Geometry: see drawing. Coordinates: mm, zero at the bounding-box minimum. A direction names the side the tool comes from. Round coordinates to 2 decimals unless told otherwise and drop trailing zeros. Write each loop counter-clockwise with the first axis right and the second up, starting at its lowest first coordinate (ties: lowest second). Pieces come first, ordered by that corner, then holes.
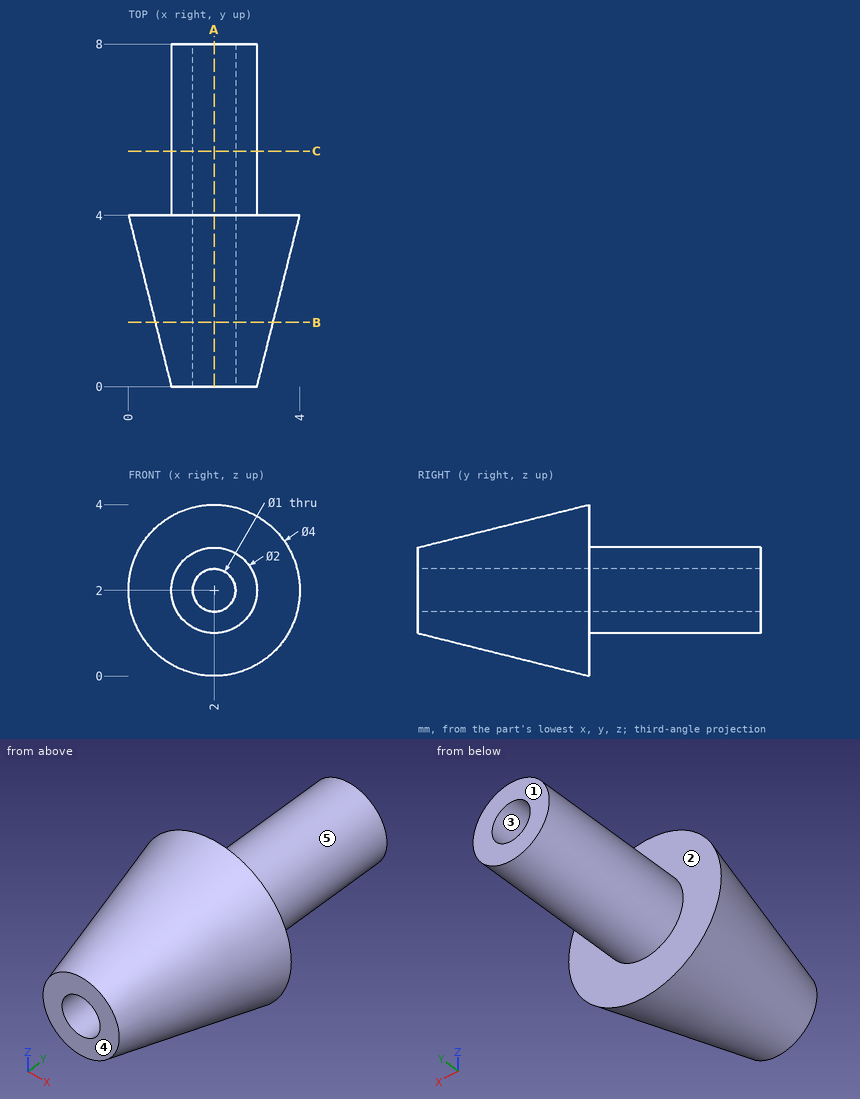
1) Reachability of the marked faces 1 and 2 from +Z, -Z, +X, -X, +Y, -Y: full face, straight path, thin tool, end or side. Return the list, or none.
Taken from the geometry:
face 1: +Z, -Z, +X, -X, +Y
face 2: +Y
2) Section query A-A on x = 2. Return the cut outline in (y, z).
Taken from the geometry:
outline: (0, 1) - (4, 0) - (4, 1) - (8, 1) - (8, 1.5) - (0, 1.5) - close; (0, 2.5) - (8, 2.5) - (8, 3) - (4, 3) - (4, 4) - (0, 3) - close
3) Contact query for flat-ended pins moving along their axis: P1, Ø1, axis at x = 1.5, y = 7, coming from the -Z side; P2, Ø1.5, axis at x = 0.5, y = 4.5, coming from the +Z side. Output: stop coordinate, or through.
Taken from the geometry:
P1: stops at z = 1
P2: stops at z = 3.76
4) Section query C-C on y = 5.5. Return the cut outline in (x, z).
Taken from the geometry:
outline: circle Ø2 at (2, 2); hole circle Ø1 at (2, 2)
5) Material intervals for line 1 (Z direction, x = 2, y = 4.25); line 2 (X direction, y = 5.25, z = 2.3); line 3 (X direction, y = 0.5, z = 1.8), sorted ascending.
Taken from the geometry:
line 1: z = 1 to 1.5, 2.5 to 3
line 2: x = 1.05 to 1.6, 2.4 to 2.95
line 3: x = 0.89 to 1.54, 2.46 to 3.11
6) Pull-direction query (Z, two-part tool) for the marked faces 3, 4 and 5; classes: released by +Z, released by -Z, zero draft, split by the parting line, or undercut.
Taken from the geometry:
face 3: undercut
face 4: zero draft
face 5: split by the parting line
7) Section query B-B on y = 1.5. Return the cut outline in (x, z) (3 decimals), then the cut area to 3 significant figures.
Taken from the geometry:
outline: circle Ø2.75 at (2, 2); hole circle Ø1 at (2, 2)
area: 5.15 mm2
